Can you work these out from the model? Positions are in its coordinate system, mm. Face numbers are marked on the shaded views. A direction names the side the tool comes from. Give positions to 0.01 mm unless a question says otherwise; leave off trailing zeros. Write each loop counter-clockwise with the first axis right and the second up, starting at its lowest first coordinate (ties: lowest second). Pieces come first, ordered by that corner, then holes.
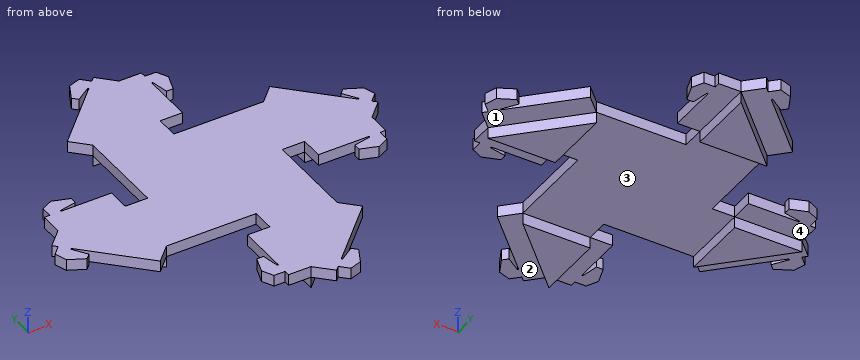
```python
from build123d import *

# Parameters (mm, degrees)
F0_W     = 152.4
F0_H     = 152.4
F0_W_2   = 50.8
F0_H_2   = 50.8
F1_DEPTH = 25.4
F2_DEPTH = 25.4


with BuildPart() as f1:
    # F0 (on Top) → F1 (new body)
    with BuildSketch(Plane.XY):
        with Locations((-76.2, -76.2)):
            Rectangle(F0_W, F0_H)
        with Locations((-76.2, 76.2)):
            Rectangle(F0_W, F0_H)
        with Locations((76.2, -76.2)):
            Rectangle(F0_W, F0_H)
        with Locations((76.2, 76.2)):
            Rectangle(F0_W, F0_H)
        with Locations((-177.8, -76.2)):
            Rectangle(F0_W_2, F0_H)
        with Locations((-76.2, 177.8)):
            Rectangle(F0_W, F0_H_2)
        with Locations((76.2, -177.8)):
            Rectangle(F0_W, F0_H_2)
        with Locations((177.8, 76.2)):
            Rectangle(F0_W_2, F0_H)
        Polygon((-355.6, 0), (-203.2, 0), (-203.2, 50.8), (-317.5, 50.8), (-342.9, 50.8), (-355.6, 50.8), align=None)
        Polygon((-203.2, -152.4), (-203.2, 0), (-355.6, 0), align=None)
        Polygon((-152.4, 203.2), (0, 203.2), (0, 355.6), align=None)
        Polygon((0, 355.6), (0, 203.2), (50.8, 203.2), (50.8, 317.5), (50.8, 342.9), (50.8, 355.6), align=None)
        Polygon((0, -355.6), (0, -203.2), (-50.8, -203.2), (-50.8, -317.5), (-50.8, -342.9), (-50.8, -355.6), align=None)
        Polygon((152.4, -203.2), (0, -203.2), (0, -355.6), align=None)
        Polygon((355.6, 0), (203.2, 0), (203.2, -50.8), (317.5, -50.8), (342.9, -50.8), (355.6, -50.8), align=None)
        Polygon((203.2, 152.4), (203.2, 0), (355.6, 0), align=None)
        Polygon((-188.3210244843, 239.1210244843), (-152.4, 203.2), (0, 355.6), (-35.9210244843, 391.5210244843), (-44.9012806053, 382.5407683632), (-62.8617928475, 364.5802561211), align=None)
        Polygon((-203.2, -152.4), (-355.6, 0), (-391.5210244843, -35.9210244843), (-382.5407683632, -44.9012806053), (-364.5802561211, -62.8617928475), (-239.1210244843, -188.3210244843), align=None)
        Polygon((239.1210244843, 188.3210244843), (203.2, 152.4), (355.6, 0), (391.5210244843, 35.9210244843), (382.5407683632, 44.9012806053), (364.5802561211, 62.8617928475), align=None)
        Polygon((152.4, -203.2), (0, -355.6), (35.9210244843, -391.5210244843), (44.9012806053, -382.5407683632), (62.8617928475, -364.5802561211), (188.3210244843, -239.1210244843), align=None)
        Polygon((-342.9, 50.8), (-317.5, 50.8), (-317.5, 53.34), (-279.4, 60.96), (-279.4, 76.2), (-317.5, 88.9), (-342.9, 76.2), align=None)
        Polygon((50.8, 342.9), (50.8, 317.5), (53.34, 317.5), (60.96, 279.4), (76.2, 279.4), (88.9, 317.5), (76.2, 342.9), align=None)
        Polygon((-50.8, -342.9), (-50.8, -317.5), (-53.34, -317.5), (-60.96, -279.4), (-76.2, -279.4), (-88.9, -317.5), (-76.2, -342.9), align=None)
        Polygon((342.9, -50.8), (317.5, -50.8), (317.5, -53.34), (279.4, -60.96), (279.4, -76.2), (317.5, -88.9), (342.9, -76.2), align=None)
        Polygon((-64.6578440717, 366.3763073453), (-62.8617928475, 364.5802561211), (-44.9012806053, 382.5407683632), (-62.8617928475, 400.5012806053), (-89.8025612107, 391.5210244843), align=None)
        Polygon((-364.5802561211, -62.8617928475), (-382.5407683632, -44.9012806053), (-400.5012806053, -62.8617928475), (-391.5210244843, -89.8025612107), (-366.3763073453, -64.6578440717), align=None)
        Polygon((366.3763073453, 64.6578440717), (364.5802561211, 62.8617928475), (382.5407683632, 44.9012806053), (400.5012806053, 62.8617928475), (391.5210244843, 89.8025612107), align=None)
        Polygon((62.8617928475, -364.5802561211), (44.9012806053, -382.5407683632), (62.8617928475, -400.5012806053), (89.8025612107, -391.5210244843), (64.6578440717, -366.3763073453), align=None)
        Polygon((-96.9867661075, 344.8236926547), (-64.6578440717, 366.3763073453), (-89.8025612107, 391.5210244843), (-107.7630734528, 355.6), align=None)
        Polygon((-344.8236926547, -96.9867661075), (-366.3763073453, -64.6578440717), (-391.5210244843, -89.8025612107), (-355.6, -107.7630734528), align=None)
        Polygon((344.8236926547, 96.9867661075), (366.3763073453, 64.6578440717), (391.5210244843, 89.8025612107), (355.6, 107.7630734528), align=None)
        Polygon((96.9867661075, -344.8236926547), (64.6578440717, -366.3763073453), (89.8025612107, -391.5210244843), (107.7630734528, -355.6), align=None)
    extrude(amount=F1_DEPTH)

    # F0 (on Top) → F2 (join)
    with BuildSketch(Plane.XY):
        Polygon((203.2, 152.4), (203.2, 0), (355.6, 0), align=None)
        Polygon((-152.4, 203.2), (0, 203.2), (0, 355.6), align=None)
        Polygon((-203.2, -152.4), (-203.2, 0), (-355.6, 0), align=None)
        Polygon((152.4, -203.2), (0, -203.2), (0, -355.6), align=None)
    extrude(amount=-F2_DEPTH)


solid = f1.part
```
1) Suppose I cut it at C-C on x = -173.5. Write out the boundary of the cut face in (y, z).
Values follow:
outline: (-152.4, 0) - (0, 0) - (0, 25.4) - (-152.4, 25.4) - close; (224.3, 0) - (253.94, 0) - (253.94, 25.4) - (224.3, 25.4) - close
2) Suppose I cut it at D-D on x = 143. Write out the boundary of the cut face in (y, z), plus the area to 3 significant figures.
Values follow:
outline: (-284.44, 0) - (-212.6, 0) - (-212.6, -25.4) - (-203.2, -25.4) - (-203.2, 0) - (152.4, 0) - (152.4, 25.4) - (-284.44, 25.4) - close
area: 11,300 mm2
3) Suppose I cut it at A-A on y = 17.5. Write out the boundary of the cut face in (x, z), plus the area to 3 significant figures.
Values follow:
outline: (-355.6, 0) - (-203.2, 0) - (-203.2, 25.4) - (-355.6, 25.4) - close; (-152.4, 0) - (203.2, 0) - (203.2, -25.4) - (338.1, -25.4) - (338.1, 0) - (373.1, 0) - (373.1, 25.4) - (-152.4, 25.4) - close
area: 20,600 mm2
4) Suppose I cut it at B-B on z = -9. Write out the boundary of the cut face in (x, y).
Values follow:
outline: (-355.6, 0) - (-203.2, -152.4) - (-203.2, 0) - close; (-152.4, 203.2) - (0, 203.2) - (0, 355.6) - close; (0, -355.6) - (152.4, -203.2) - (0, -203.2) - close; (203.2, 0) - (355.6, 0) - (203.2, 152.4) - close
5) For pin 1 Ø1 at (y, z) = (-27, -6.5) entering from +X; pin 2 Ø20.5 at (y, z) = (182, 17.5) entering from +X; pin 3 Ø0.8 at (x, z) = (-52.5, 11.5) entering from +Y, each with a flat end and sliding along its axis, tell me the tip position at first contact or that it passes through.
Values follow:
pin 1: stops at x = -203.2
pin 2: stops at x = 255.69
pin 3: stops at y = 390.54
6) Please list where these lines run through material, in increasing order: L1, parallel to X at y = -67.5, z = 3.5; L2, parallel to Z at x = 30, y = 41; L3, parallel to X at y = 3, z = 11.5.
Values follow:
L1: x = -398.96 to -364.48, -359.94 to 152.4, 279.4 to 342.9
L2: z = 0 to 25.4
L3: x = -355.6 to -203.2, -152.4 to 358.6
7) For the marked faces 1, 2, 3 and 4, which set-ups out of +Z, -Z, +X, -X, +Y, -Y let a thin tool reach every point of the face, with its end or its side?
Values follow:
face 1: -Z, +X, +Y
face 2: -Z, +X, -Y
face 3: -Z
face 4: -Z, -X, +Y
